Geometry check sheet. Reference: drawing and pictorial views, mm from the part's lowest x, y, z. Give positions to 0.01 mm unless a question says otherwise; leave off trailing zeros. Loops run counter-clockwise (first coordinate to the right, second up) from the corner with the lowest first, then second, coordinate; pieces in that order, holes last. Notation, with made-up numbers: (16, -40) - (73, -40) arc R16 cw to (73, -23) - close; hole circle Ø6 at (-38, 36). An arc over 180 degrees is marked (long way). Put each result on its own line as item: value. Start each with the question number.
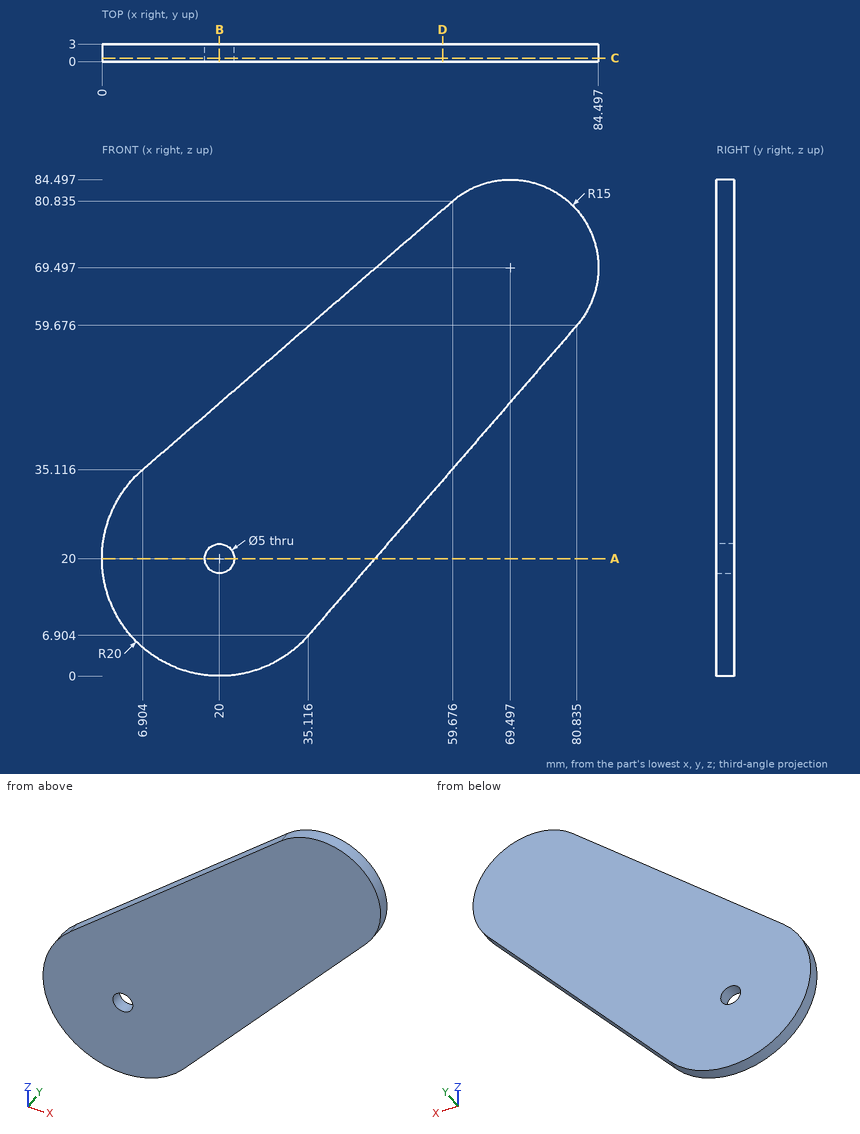
1) Scan lines: line 1 along Z through (x, y) = (22, 2.4) (1 decimal); line 2 along X through (y, z) = (2.25, 20); line 3 along X through (y, z) = (2.15, 5). Record each from-to range of solid material in increasing order. Write a range as from..to.
2) Section check A-A, the plane z = 20. Enter the section's corners in (x, y).
3) Depth check by flat-ended pin: P1, Ø8, axis at x = 53.5, z = 49, coming from the -Y side; P2, Ø1, axis at x = 21, y = 2, coming from the -Z side; P3, Ø1, axis at y = 1.5, z = 38, coming from the -X side (1 decimal); P4, Ø1, axis at y = 2.5, z = 56, coming from the -X side. Enter the tip coordinate at first touch or a pass-through.
4) Section check C-C, the plane y = 0.6. Enter the section's corners in (x, z) (1 decimal).
5) Section check D-D, the plane x = 58. Enter the section's corners in (y, z).
6) Section check B-B, the plane x = 20. Enter the section's corners in (y, z), plus the area to 3 significant figures.
Results are:
1. line 1: z = 0.1..18.5, 21.5..48.2
1. line 2: x = 0..17.5, 22.5..46.46
1. line 3: x = 6.77..33.23
2. outline: (0, 0) - (17.5, 0) - (17.5, 3) - (0, 3) - close; (22.5, 0) - (46.46, 0) - (46.46, 3) - (22.5, 3) - close
3. P1: stops at y = 0
3. P2: stops at z = 0.01
3. P3: stops at x = 9.7
3. P4: stops at x = 30.43
4. outline: (6.9, 35.1) arc R20 ccw (long way) to (35.1, 6.9) - (80.8, 59.7) arc R15 ccw to (59.7, 80.8) - close; hole circle Ø5 at (20, 20)
5. outline: (0, 33.32) - (3, 33.32) - (3, 79.38) - (0, 79.38) - close
6. outline: (0, 0) - (3, 0) - (3, 17.5) - (0, 17.5) - close; (0, 22.5) - (3, 22.5) - (3, 46.46) - (0, 46.46) - close
6. area: 124 mm2
